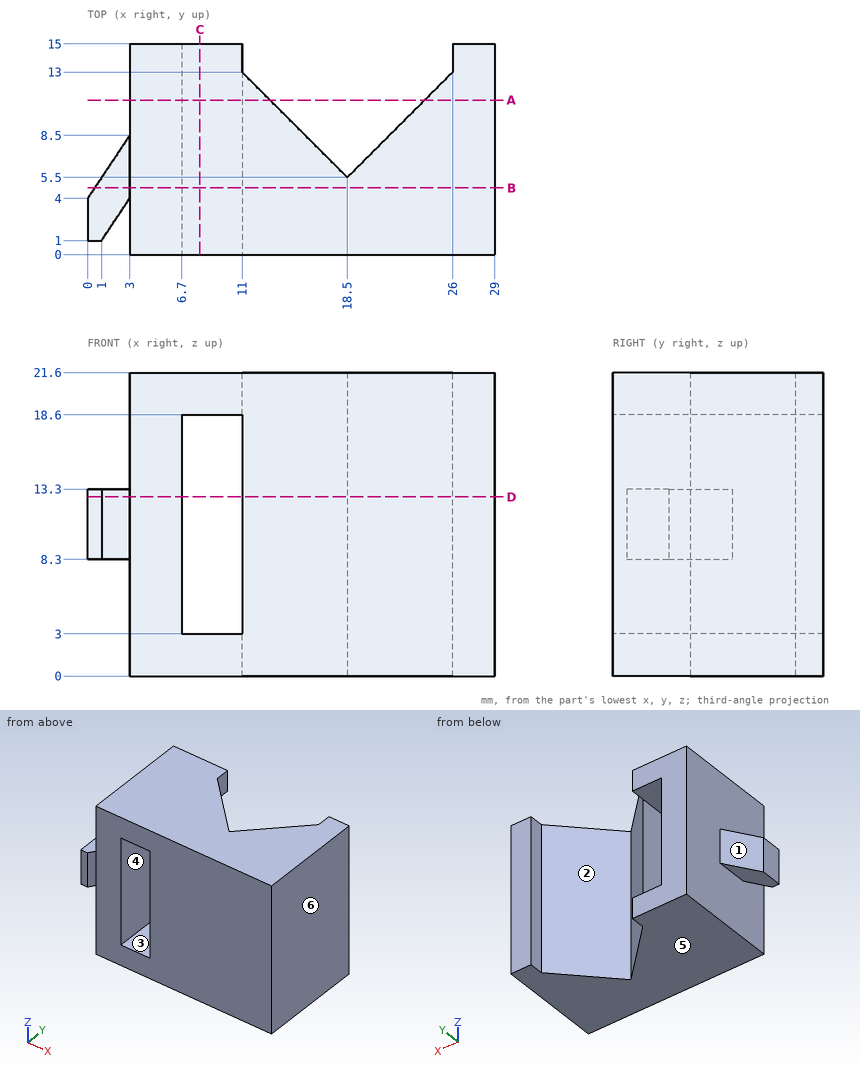
Answer from the drawing. Dimensions are ordinates in mm from the lowest x, y and z of the part. A direction names the side the tool comes from. Coordinates: 2 decimals unless noted, no trailing zeros. Write each loop counter-clockwise with the first axis right and the second up, starting at its lowest first coordinate (ties: lowest second). Pieces come first, ordered by that corner, then holes. Notation, with made-up numbers: (8.25, 11.25) - (48.25, 11.25) arc R30 ccw to (48.25, 43.25) - close; hole circle Ø8 at (40, -5.5). An arc over 180 degrees is marked (long way). Return JSON: item names as keys, results as strings. Group by question number.
Q1. Flat-ended cylindrical pins translate along their axes: pin 1 Ø2 at (y, z) = (14.5, 13.5) entering from -X; pin 2 Ø1.1 at (x, z) = (0.5, 11) entering from -Y. Find the tip coordinate at first contact, or state that the pin passes through.
Q2. Find the intervals of material crossed by line 1 along X through (y, z) = (1.75, 6.25); line 2 along X through (y, z) = (10, 17.25); line 3 along X through (y, z) = (8.75, 8.75), in increasing order. Write a range as [from, to].
Q3. Which of the six approach directions +Z, -Z, +X, -X, +Y, -Y give full straight-line access (tool end or side, diameter ignored) to the marked faces 1, 2 and 3?
Q4. The part is cut by section D-D on z = 12.75. Write down the section's boundary in (x, y), and give its area (3 significant figures).
Q5. The part is cut by section C-C on x = 8. Write down the section's boundary in (y, z).
Q6. The part is cut by section B-B on y = 4.75. Write down the section's boundary in (x, z), and give its area (3 significant figures).
Q7. The part is cut by section A-A on y = 11. Write down the section's boundary in (x, z).
Q8. For a pull along X with two mould halves and no side action, classify the marked faces 4, 5 and 6 as +X half, -X half, draft (parallel to the pull), parting line (faces both ways), or undercut.
Evaluation:
{
 "1": {"pin 1": "stops at x = 3", "pin 2": "stops at y = 1"},
 "2": {"line 1": "x = [3, 6.7], [11, 29]", "line 2": "x = [3, 6.7], [11, 14], [23, 29]", "line 3": "x = [3, 6.7], [11, 15.25], [21.75, 29]"},
 "3": {"face 1": "+Z, -Z, -X, +Y", "face 2": "+Z, -Z, +Y", "face 3": "+Y, -Y"},
 "4": {"outline": "(0, 1) - (1, 1) - (3, 4) - (3, 0) - (6.7, 0) - (6.7, 15) - (3, 15) - (3, 8.5) - (0, 4) - close; (11, 0) - (29, 0) - (29, 15) - (26, 15) - (26, 13) - (18.5, 5.5) - (11, 13) - close", "area": "252 mm2"},
 "5": {"outline": "(0, 0) - (15, 0) - (15, 3) - (0, 3) - close; (0, 18.6) - (15, 18.6) - (15, 21.6) - (0, 21.6) - close"},
 "6": {"outline": "(0.5, 8.3) - (3, 8.3) - (3, 0) - (29, 0) - (29, 21.6) - (3, 21.6) - (3, 13.3) - (0.5, 13.3) - close; hole (6.7, 3) - (11, 3) - (11, 18.6) - (6.7, 18.6) - close", "area": "507 mm2"},
 "7": {"outline": "(3, 0) - (13, 0) - (13, 21.6) - (3, 21.6) - close; (24, 0) - (29, 0) - (29, 21.6) - (24, 21.6) - close; hole (6.7, 3) - (11, 3) - (11, 18.6) - (6.7, 18.6) - close"},
 "8": {"face 4": "undercut", "face 5": "draft", "face 6": "+X half"}
}
